from build123d import *

# Parameters (mm, degrees)
F1_DEPTH      = 228.6
F2_W          = 12.7
F2_H          = 6.35
F3_DEPTH      = 11.938
F3_DEPTH_BACK = 25.4
F4_W          = 6.35
F4_H          = 12.7
F5_DEPTH      = 12.7
F6_R          = 2.579688
F7_DEPTH      = 12.7
F8_R          = 2.579688
F9_DEPTH      = 12.7


with BuildPart() as f1:
    # F0 (on Front) → F1 (new body)
    with BuildSketch(Plane.XZ):
        with BuildLine():
            ThreePointArc((10.071912, -2.38125), (9.37446, -0.697452), (7.690662, 0))
            Line((7.690662, 0), (-0.246838, 0))
            ThreePointArc((-0.246838, 0), (-1.930636, -0.697452), (-2.628088, -2.38125))
            Line((-2.628088, -2.38125), (-2.628088, -10.31875))
            ThreePointArc((-2.628088, -10.31875), (-1.930636, -12.002548), (-0.246838, -12.7))
            Line((-0.246838, -12.7), (7.690662, -12.7))
            ThreePointArc((7.690662, -12.7), (9.37446, -12.002548), (10.071912, -10.31875))
            Line((10.071912, -10.31875), (10.071912, -2.38125))
        make_face()
        with BuildLine():
            Line((0.546912, -1.5875), (6.896912, -1.5875))
            ThreePointArc((6.896912, -1.5875), (8.019444, -2.052468), (8.484412, -3.175))
            Line((8.484412, -3.175), (8.484412, -9.525))
            ThreePointArc((8.484412, -9.525), (8.019444, -10.647532), (6.896912, -11.1125))
            Line((6.896912, -11.1125), (0.546912, -11.1125))
            ThreePointArc((0.546912, -11.1125), (-0.57562, -10.647532), (-1.040588, -9.525))
            Line((-1.040588, -9.525), (-1.040588, -3.175))
            ThreePointArc((-1.040588, -3.175), (-0.57562, -2.052468), (0.546912, -1.5875))
        make_face(mode=Mode.SUBTRACT)
    extrude(amount=F1_DEPTH)

    # F2 (on Right) → F3 (cut, two sides)
    with BuildSketch(Plane.YZ) as f3_sk:
        with Locations((-215.9, -3.175)):
            Rectangle(F2_W, F2_H)
        with Locations((-12.7, -3.175)):
            Rectangle(F2_W, F2_H)
    extrude(amount=F3_DEPTH, mode=Mode.SUBTRACT)
    extrude(f3_sk.sketch, amount=-F3_DEPTH_BACK, mode=Mode.SUBTRACT)

    # F4 (on Top) → F5 (cut)
    with BuildSketch(Plane.XY):
        with Locations((0.546912, -114.3)):
            Rectangle(F4_W, F4_H)
    extrude(amount=-F5_DEPTH, mode=Mode.SUBTRACT)

    # F6 (on Top) → F7 (cut)
    with BuildSketch(Plane.XY):
        with Locations((3.721912, -12.7)):
            Circle(F6_R)
        with Locations((3.721912, -215.9)):
            Circle(F6_R)
    extrude(amount=-F7_DEPTH, mode=Mode.SUBTRACT)

    # F8 (on Right) → F9 (cut)
    with BuildSketch(Plane.YZ):
        with Locations((-114.3, -6.35)):
            Circle(F8_R)
    extrude(amount=F9_DEPTH, mode=Mode.SUBTRACT)


solid = f1.part
The listing builds one solid part. Answer for the finished solid, in the listing's coordinates (mm). A direction names the side the tool comes from. Round coordinates to 2 decimals unless told otherwise and drop trailing zeros. Loops run counter-clockwise (first coordinate to the right, second up) from the corner with the lowest first, then second, coordinate; pieces in that order, holes last. Notation, with made-up numbers: M -7,84.25 L 12,84.25 A27 cw 12,118.25 Z; hole C 17,76 d5. An arc over 180 degrees is marked long. Write each question's results on one line, items separated by ' | '. Start each with the question number.
1) Each of these flat-tipped pins is pushed along its axis until it touches: pin 1 (1.7 mm diameter, centred on x = -1.5, y = -218.5, fed in from +Z); pin 2 (1.3 mm diameter, centred on y = -115, z = -12, fed in from -X); pin 3 (3 mm diameter, centred on x = 6, z = -4, fed in from +Y); pin 4 (6 mm diameter, centred on x = 3.72, y = -215.9, fed in from +Z). Where does it stop, or does it pass through?
2) Which of the six approach directions +Z, -Z, +X, -X, +Y, -Y give full straight-line access (tool end or side, diameter ignored) to faces 1 (the flat face through (4, -228.6, -12)), 2 (the flat face through (4, -113, -11.112)), 3 (the flat face through (4, -3, 0)), 4 (the flat face through (4, -19.05, -1)), 5 (the flat face through (-2, -120.65, -6))?
3) Find section A-A on y = -114.3. Write down the section's boundary in (x, z) (1 decimal).
4) Straight lines are drawn through the part: probe 1 along Y at (x, z) = (-2, -4.75); probe 2 along X at (y, z) = (-80.5, -3.25); probe 3 along Z at (x, y) = (4.75, -196). For each, find the intervals that lie inside material, in ascending order.
5) Determine the mould class of faces 6 (the flat face through (4, -225, 0)), 7 (the cylindrical face through (9.267, -116.877, -6.237)), 8 (the flat face through (4, 0, -12)) for opening direction Y: pulls with the +Y half, pulls with the -Y half, needs draft (parallel to the pull), parting line crosses it, or undercut.
Final values:
1) pin 1: z = -6.35 | pin 2: x = 3.72 | pin 3: through | pin 4: z = -11.11
2) face 1: +Z, -Z, +X, -X, -Y | face 2: +Y, -Y | face 3: +Z, +X, -X, +Y, -Y | face 4: +Z, +X, -X | face 5: +Z, -Z, -X
3) outline: M 3.7,-12.7 L 7.7,-12.7 A2.4 ccw 10.1,-10.3 L 10.1,-8.9 L 8.5,-8.9 L 8.5,-9.5 A1.6 cw 6.9,-11.1 L 3.7,-11.1 Z; M 3.7,-1.6 L 6.9,-1.6 A1.6 cw 8.5,-3.2 L 8.5,-3.8 L 10.1,-3.8 L 10.1,-2.4 A2.4 ccw 7.7,0 L 3.7,0 Z
4) probe 1: -228.6 to -222.25, -209.55 to -120.65, -107.95 to -19.05, -6.35 to 0 | probe 2: -2.63 to -1.04, 8.48 to 10.07 | probe 3: -12.7 to -11.11, -1.59 to 0
5) face 6: needs draft | face 7: undercut | face 8: pulls with the +Y half
